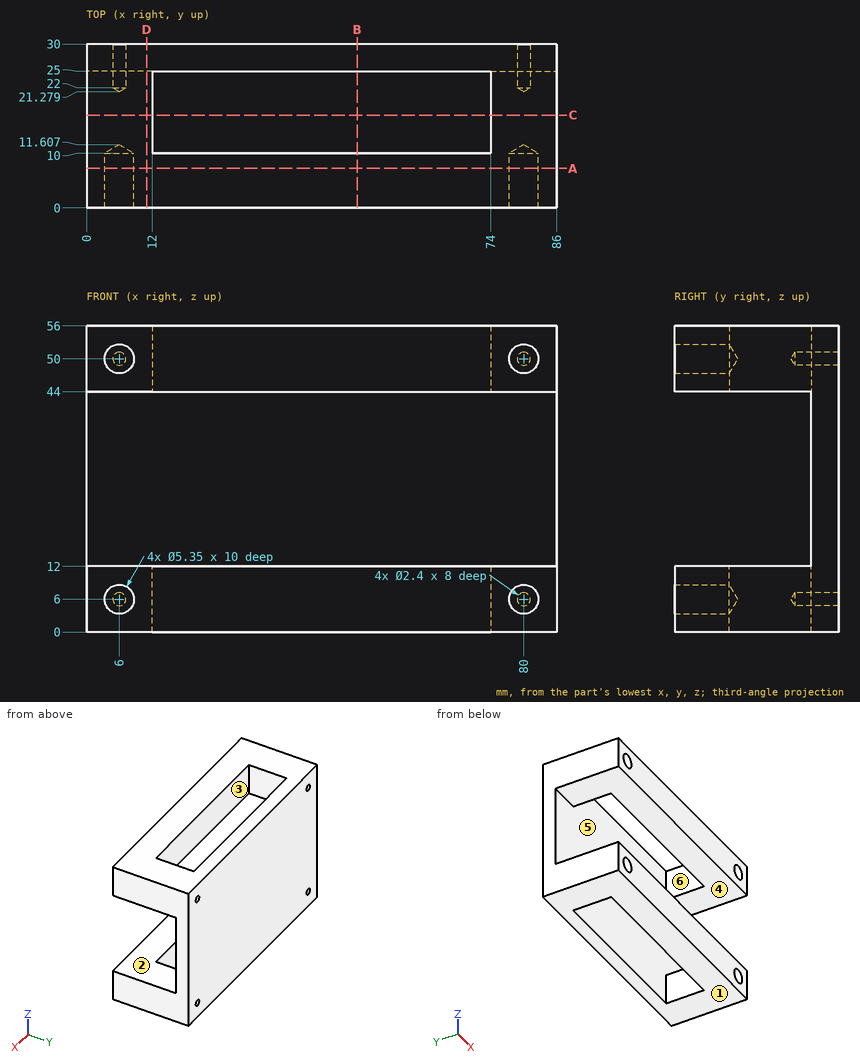
Part print with two shaded views. Sizes in mm from the minimum x, y, z corner. A direction names the side the tool comes from. Coordinates: 2 decimals unless noted, no trailing zeros. Write each loop counter-clockwise with the first axis right and the second up, starting at its lowest first coordinate (ties: lowest second). Pieces come first, ordered by that corner, then holes. Notation, with made-up numbers: (66.5, 50.25) - (75.5, 50.25) arc R18 cw to (75.5, 78.25) - close; hole circle Ø5 at (43, 13). An arc over 180 degrees is marked (long way). Use a Markdown table: item, result. Add a question column.
Item 1: Two-plate mould, pull along Z, no slides. Class the marked faces 1, 2 and 3: pulls with the +Z half, pulls with the -Z half, needs draft (parallel to the pull), parting line crosses it, or undercut.
Item 2: Band-saw the part on A-A, the plane y = 7.25. Give the number of separate pieces and of enclosed holes in the cut face, and give its area (3 significant figures).
Item 3: Band-saw the part on D-D, the plane x = 11. Write the cut outline in (y, z), and give its area (3 significant figures).
Item 4: Band-saw the part on C-C, the plane y = 17. Write the cut outline in (x, z).
Item 5: Band-saw the part on B-B, the plane x = 49.5. Write the cut outline in (y, z).
Item 6: Drill centre lines: line 1 along X through (y, z) = (7, 6) (1 decimal); line 2 along Z through (x, y) = (6, 26.75); line 3 along Z through (x, y) = (6, 4.25) (1 decimal). Where is each one in solid material? Low to high.
Item 7: Drop flat-ended pins along their axis: pin 1 (2 mm diameter, centred on x = 77, z = 27.5, fed in from -Y); pin 2 (3 mm diameter, centred on x = 6, z = 50, fed in from -Y); pin 3 (1.4 mm diameter, centred on x = 80, z = 50, fed in from +Y). Give the stop position or say it passes through.
Item 8: 3-axis set-ups, long thin cutter, end or side, ignore diameter. For the marked faces 4, 5 and 6: which of +Z, -Z, +X, -X, +Y, -Y reach the whole face in a straight line?
A:
| question | item | result |
|---|---|---|
| 1 | face 1 | pulls with the -Z half |
| 1 | face 2 | undercut |
| 1 | face 3 | needs draft |
| 2 | separate pieces | 2 |
| 2 | enclosed holes | 4 |
| 2 | area | 1,970 mm² |
| 3 | outline | (0, 0) - (30, 0) - (30, 56) - (0, 56) - (0, 44) - (25, 44) - (25, 12) - (0, 12) - close |
| 3 | area | 880 mm² |
| 4 | outline | (0, 0) - (12, 0) - (12, 12) - (0, 12) - close; (0, 44) - (12, 44) - (12, 56) - (0, 56) - close; (74, 0) - (86, 0) - (86, 12) - (74, 12) - close; (74, 44) - (86, 44) - (86, 56) - (74, 56) - close |
| 5 | outline | (0, 0) - (10, 0) - (10, 12) - (0, 12) - close; (0, 44) - (10, 44) - (10, 56) - (0, 56) - close; (25, 0) - (30, 0) - (30, 56) - (25, 56) - close |
| 6 | line 1 | x = 0 to 3.3, 8.7 to 77.3, 82.7 to 86 |
| 6 | line 2 | z = 0 to 4.8, 7.2 to 48.8, 51.2 to 56 |
| 6 | line 3 | z = 0 to 3.3, 8.7 to 12, 44 to 47.3, 52.7 to 56 |
| 7 | pin 1 | stops at y = 25 |
| 7 | pin 2 | stops at y = 10.71 |
| 7 | pin 3 | stops at y = 21.7 |
| 8 | face 4 | +X, -X, -Y |
| 8 | face 5 | none |
| 8 | face 6 | +Z, -Z |
